Input: part model. Units: mm. Frame: model coordinates. A direction names the side the tool comes from. Round coordinates to 2 decimals unless told otherwise and drop trailing zeros. Loops run counter-clockwise (first coordinate to the right, second up) from the corner with the lowest first, then second, coordinate; pieces in that order, holes last. Notation, with made-up numbers: (73.25, -16) -> (124.25, -16) arc R20 cw to (124.25, -5) -> close; hole circle Ø1 at (69, 55). An arc over 180 degrees is marked (long way). Answer as a JSON object with one key per item and string values.
```python
from build123d import *

# Parameters (mm, degrees)
F0_W     = 32
F0_H     = 16
F1_DEPTH = 8
F3_R     = 2.5
F4_DEPTH = 2
F5_T     = -1


# Not quite as in the source:
# - the program builds the solid bodies; features that only make, move or delete a surface that nothing else refers to are left out


with BuildPart() as f1:
    # F0 (on Top) → F1 (new body)
    with BuildSketch(Plane.XY):
        with Locations((0.0749295065, 8)):
            Rectangle(F0_W, F0_H)
    extrude(amount=F1_DEPTH)

    # F3 (on offset) → F4 (join)
    with BuildSketch(Plane.XY.offset(8)):
        with Locations((-8.4686602995, 10.8479883277)):
            Circle(F3_R)
        with Locations((-2.7646990493, 10.774385184)):
            Circle(F3_R)
        with Locations((3.3415844664, 10.774385184)):
            Circle(F3_R)
        with Locations((8.8161835447, 10.8445733786)):
            Circle(F3_R)
        with Locations((8.8161835447, 5.0892247818)):
            Circle(F3_R)
        with Locations((3.4117714968, 5.0892247818)):
            Circle(F3_R)
        with Locations((-2.7646990493, 5.2295993082)):
            Circle(F3_R)
        with Locations((-8.4498599172, 5.2295993082)):
            Circle(F3_R)
    extrude(amount=F4_DEPTH)

    # F5
    f5_openings = [f1.faces().sort_by_distance(p)[0] for p in [
        (0.07493, 8, 0),
    ]]
    offset(amount=F5_T, openings=f5_openings, kind=Kind.INTERSECTION)


solid = f1.part
```
1) Section B-B, the plane z = 4.25. Output: boundary loops of the cut face in (x, y), plus the area to 3 significant figures.
Output:
{"outline": "(-15.93, 0) -> (16.07, 0) -> (16.07, 16) -> (-15.93, 16) -> close; hole (-14.93, 1) -> (15.07, 1) -> (15.07, 15) -> (-14.93, 15) -> close", "area": "92.0 mm^2"}
2) Contact query for flat-ended pins moving along their axis: P1, Ø2.5, axis at x = 3.34, y = 10.77, coming from the -Z side; P2, Ø3.5, axis at x = -8.5, y = 11, coming from the -Z side. Output: stop coordinate, or through.
Output:
{"P1": "stops at z = 9", "P2": "stops at z = 7"}
3) Section A-A, the plane x = -12. Output: boundary loops of the cut face in (y, z), plus the area to 3 significant figures.
Output:
{"outline": "(0, 0) -> (1, 0) -> (1, 7) -> (15, 7) -> (15, 0) -> (16, 0) -> (16, 8) -> (0, 8) -> close", "area": "30.0 mm^2"}
4) Section D-D, the plane x = 3. Output: boundary loops of the cut face in (y, z).
Output:
{"outline": "(0, 0) -> (1, 0) -> (1, 7) -> (3.65, 7) -> (3.65, 9) -> (6.53, 9) -> (6.53, 7) -> (9.31, 7) -> (9.31, 9) -> (12.23, 9) -> (12.23, 7) -> (15, 7) -> (15, 0) -> (16, 0) -> (16, 8) -> (13.25, 8) -> (13.25, 10) -> (8.3, 10) -> (8.3, 8) -> (7.56, 8) -> (7.56, 10) -> (2.62, 10) -> (2.62, 8) -> (0, 8) -> close"}
5) Draft query along Y for faces 4 (the face through (-9, 11, 10)), 5 (the face through (-9.574, 11.862, 7.986)), 6 (the face through (0, 0, 4)). Return one class per face: +Y half, -Y half, draft (parallel to the pull), parting line (faces both ways), or undercut.
Output:
{"face 4": "draft", "face 5": "undercut", "face 6": "-Y half"}
6) Ray query, probe 1 along X at (y, z) = (5.5, 2.25); probe 2 along Y at (x, z) = (-9.5, 3.25); probe 3 along X at (y, z) = (4.75, 7.5). Return the intervals inside material, ascending.
Output:
{"probe 1": "x = -15.93 to -14.93, 15.07 to 16.07", "probe 2": "y = 0 to 1, 15 to 16", "probe 3": "x = -15.93 to -9.87, -7.03 to -4.19, -1.34 to 1.95, 4.87 to 7.36, 10.28 to 16.07"}
7) Section C-C, the plane y = 14.25. Output: boundary loops of the cut face in (x, z), plus the area to 3 significant figures.
Output:
{"outline": "(-15.93, 0) -> (-14.93, 0) -> (-14.93, 7) -> (15.07, 7) -> (15.07, 0) -> (16.07, 0) -> (16.07, 8) -> (-15.93, 8) -> close", "area": "46.0 mm^2"}
8) Reachability of faces 1 (the face through (3, 11, 9)), 2 (the face through (3, 11, 10)), 3 (the face through (0.914, 5.199, 8.986)) from +Z, -Z, +X, -X, +Y, -Y: full face, straight path, thin tool, end or side. Return the list, or none.
Output:
{"face 1": "-Z", "face 2": "+Z, +X, -X, +Y, -Y", "face 3": "+Z"}
